Geometry: final body of the model. Coordinates: model frame, mm. A direction names the side the tool comes from. Coordinates: 2 decimals unless noted, no trailing zeros. Write each loop counter-clockwise with the first axis right and the second up, starting at its lowest first coordinate (ties: lowest second). Pieces come first, ordered by that corner, then holes.
from build123d import *

# Parameters (mm, degrees)
SKETCH_1_R               = 9.25
SKETCH_1_R_2             = 2.5
EXTRUDE_1_DEPTH          = 8
SKETCH_2_R               = 2.5
CUT_EXTRUDE_1_DEPTH      = 9
CUT_EXTRUDE_2_DEPTH      = 9
SKETCH_8_R               = 9.25
SKETCH_8_R_2             = 2.5
EXTRUDE_2_DEPTH          = 8
SKETCH_9_R               = 1.75
CUT_EXTRUDE_5_DEPTH      = 56
CUT_EXTRUDE_5_DEPTH_BACK = 56
SKETCH_11_W              = 2.84011948
SKETCH_11_H              = 7
CUT_EXTRUDE_6_DEPTH      = 8
EXTRUDE_3_DEPTH          = 8
SKETCH_12_R              = 1.65
CUT_EXTRUDE_7_DEPTH      = 9
CHAMFER_2_SIZE           = 1


with BuildPart() as part:
    # Sketch 1 → Extrude 1 (new body)
    with BuildSketch(Plane.XY):
        with BuildLine():
            Line((-50, -20), (50, -20))
            ThreePointArc((50, -20), (54.789131426, -16.436739428), (52.752293578, -10.825688073))
            Line((52.752293578, -10.825688073), (11.009174312, 16.697247706))
            ThreePointArc((11.009174312, 16.697247706), (0, 20), (-11.009174312, 16.697247706))
            Line((-11.009174312, 16.697247706), (-52.752293578, -10.825688073))
            ThreePointArc((-52.752293578, -10.825688073), (-54.789131426, -16.436739428), (-50, -20))
        make_face()
        Circle(SKETCH_1_R, mode=Mode.SUBTRACT)
        with Locations((50, -15)):
            Circle(SKETCH_1_R_2, mode=Mode.SUBTRACT)
        with Locations((-50, -15)):
            Circle(SKETCH_1_R_2, mode=Mode.SUBTRACT)
    extrude(amount=EXTRUDE_1_DEPTH)

    # Sketch 2 → Cut-Extrude 1 (cut, through all)
    with BuildSketch(Plane.XY.offset(8)):
        with Locations((0, 15)):
            Circle(SKETCH_2_R)
        with Locations((-10.606601718, 10.606601718)):
            Circle(SKETCH_2_R)
        with Locations((10.606601718, 10.606601718)):
            Circle(SKETCH_2_R)
    extrude(amount=-CUT_EXTRUDE_1_DEPTH, mode=Mode.SUBTRACT)

    # Sketch 3 → Cut-Extrude 2 (cut, through all)
    with BuildSketch(Plane.XY.offset(8)):
        with BuildLine():
            Line((-44.573394495, -11.422018349), (-15.198052695, 7.946338883))
            ThreePointArc((-15.198052695, 7.946338883), (-13.864095006, 6.417668929), (-12.053948035, 5.501348633))
            ThreePointArc((-12.053948035, 5.501348633), (-12.001148515, -5.615597414), (-3.5, -12.779377919))
            Line((-3.5, -12.779377919), (-3.5, -15))
            Line((-3.5, -15), (-43.5, -15))
            ThreePointArc((-43.5, -15), (-43.774129146, -13.132238744), (-44.573394495, -11.422018349))
        make_face()
    cut_extrude_2 = extrude(amount=-CUT_EXTRUDE_2_DEPTH, mode=Mode.SUBTRACT)

    # Mirror 1: Cut-Extrude 2 across plane
    add(cut_extrude_2.mirror(Plane(origin=(0, 0, 0), x_dir=(0, 0, 1), z_dir=(1, 0, 0))), mode=Mode.SUBTRACT)

    # Sketch 8 → Extrude 2 (add)
    with BuildSketch(Plane.XY.offset(8)):
        with BuildLine():
            Line((-11.009174312, 16.697247706), (-13.527583827, 15.036757916))
            ThreePointArc((-13.527583827, 15.036757916), (-15.771645109, 11.823461278), (-15.198052695, 7.946338883))
            ThreePointArc((-15.198052695, 7.946338883), (-13.864095006, 6.417668929), (-12.053948035, 5.501348633))
            ThreePointArc((-12.053948035, 5.501348633), (-12.001148515, -5.615597414), (-3.5, -12.779377919))
            ThreePointArc((-3.5, -12.779377919), (0, -13.25), (3.5, -12.779377919))
            ThreePointArc((3.5, -12.779377919), (12.001148515, -5.615597414), (12.053948035, 5.501348633))
            ThreePointArc((12.053948035, 5.501348633), (13.864095006, 6.417668929), (15.198052695, 7.946338883))
            ThreePointArc((15.198052695, 7.946338883), (15.771645109, 11.823461278), (13.527583827, 15.036757916))
            Line((13.527583827, 15.036757916), (11.009174312, 16.697247706))
            ThreePointArc((11.009174312, 16.697247706), (0, 20), (-11.009174312, 16.697247706))
        make_face()
        Circle(SKETCH_8_R, mode=Mode.SUBTRACT)
        with Locations((-10.606601718, 10.606601718)):
            Circle(SKETCH_8_R_2, mode=Mode.SUBTRACT)
        with Locations((10.606601718, 10.606601718)):
            Circle(SKETCH_8_R_2, mode=Mode.SUBTRACT)
        with Locations((0, 15)):
            Circle(SKETCH_8_R_2, mode=Mode.SUBTRACT)
    extrude(amount=EXTRUDE_2_DEPTH)

    # Sketch 9 → Cut-Extrude 5 (cut, two sides)
    with BuildSketch(Plane(origin=(0, 0, 0), x_dir=(0, 0, -1), z_dir=(1, 0, 0))) as cut_extrude_5_sk:
        with Locations((-12, 0)):
            Circle(SKETCH_9_R)
    extrude(amount=CUT_EXTRUDE_5_DEPTH, mode=Mode.SUBTRACT)
    extrude(cut_extrude_5_sk.sketch, amount=-CUT_EXTRUDE_5_DEPTH_BACK, mode=Mode.SUBTRACT)

    # Sketch 11 → Cut-Extrude 6 (cut)
    with BuildSketch(Plane.XY.offset(16)):
        with Locations((14.199437659, 0)):
            Rectangle(SKETCH_11_W, SKETCH_11_H)
        with Locations((-14.199437659, 0)):
            Rectangle(SKETCH_11_W, SKETCH_11_H)
    extrude(amount=-CUT_EXTRUDE_6_DEPTH, mode=Mode.SUBTRACT)

    # Sketch 13 → Extrude 3 (add)
    with BuildSketch(Plane.XY.offset(8)):
        with BuildLine():
            Line((-37.875, -10), (-35, -10))
            ThreePointArc((-35, -10), (-30, -15), (-35, -20))
            Line((-35, -20), (-44.573394495, -20))
            Line((-44.573394495, -20), (-44.573394495, -11.422018349))
            Line((-44.573394495, -11.422018349), (-39.251146789, -7.912844037))
            Line((-39.251146789, -7.912844037), (-37.875, -10))
        make_face()
    extrude_3 = extrude(amount=-EXTRUDE_3_DEPTH)

    # Sketch 12 → Cut-Extrude 7 (cut, through all)
    with BuildSketch(Plane.XY.offset(8)):
        with Locations((-42, -15)):
            Circle(SKETCH_12_R)
        with Locations((-35, -15)):
            Circle(SKETCH_12_R)
    cut_extrude_7 = extrude(amount=-CUT_EXTRUDE_7_DEPTH, mode=Mode.SUBTRACT)

    # Mirror 2: Extrude 3, Cut-Extrude 7 across plane
    add(extrude_3.mirror(Plane(origin=(0, 0, 0), x_dir=(0, 0, 1), z_dir=(1, 0, 0))))
    add(cut_extrude_7.mirror(Plane(origin=(0, 0, 0), x_dir=(0, 0, 1), z_dir=(1, 0, 0))), mode=Mode.SUBTRACT)

    # Chamfer 2
    chamfer_2_edges = [part.edges().sort_by_distance(p)[0] for p in [
        (8.106601718, 10.606601718, 0),
        (-13.106601718, 10.606601718, 0),
        (-2.5, 15, 0),
        (-13.106601718, 10.606601718, 16),
        (-2.5, 15, 16),
        (8.106601718, 10.606601718, 16),
    ]]
    chamfer(chamfer_2_edges, length=CHAMFER_2_SIZE)


solid = part.part
Item 1: Material intervals for probe 1 along Y at (x, z) = (0, 5.25); probe 2 along X at (y, z) = (-7, 3.25); probe 3 along Y at (x, z) = (9.95, 12), sorted ascending.
Derived:
probe 1: y = -20 to -9.25, 9.25 to 12.5, 17.5 to 20
probe 2: x = -46.95 to -37.87, -11.25 to -6.05, 6.05 to 11.25, 37.87 to 46.95
probe 3: y = -8.75 to -1.75, 1.75 to 8.19, 13.02 to 17.35
Item 2: Set-up query: faces 1 (the flat face through (-36, -10, 4)), 2 (the cylindrical face through (-10.905, 0.526, 10.331)). Return all of +Z, -Z, +X, -X, +Y, -Y with unobstructed straight access to the full face (end or side cutting, diameter ignored); none if empty.
Derived:
face 1: +Z, -Z
face 2: +X, -X
Item 3: Section A-A, the plane x = 0. Output: boundary loops of the cut face in (y, z).
Derived:
outline: (-20, 0) - (-9.25, 0) - (-9.25, 16) - (-13.25, 16) - (-13.25, 8) - (-20, 8) - close; (9.25, 0) - (11.5, 0) - (12.5, 1) - (12.5, 15) - (11.5, 16) - (9.25, 16) - close; (17.5, 1) - (18.5, 0) - (20, 0) - (20, 16) - (18.5, 16) - (17.5, 15) - close
Item 4: Pin query (flat end, axial travel): pin 1 (1 mm diameter, centred on y = 15, z = 8.5, fed in from +X); pin 2 (4 mm diameter, centred on x = 42, y = -15, fed in from +Z); pin 3 (2 mm diameter, centred on y = 0, z = 12, fed in from -X); pin 4 (1 mm diameter, centred on x = 31, y = -14, fed in from -Z). Return the tip coordinate at first contact, or that it passes through.
Derived:
pin 1: stops at x = 14.21
pin 2: stops at z = 8
pin 3: passes through
pin 4: stops at z = 0
Item 5: Section C-C, the plane x = 32. Output: boundary loops of the cut face in (y, z).
Derived:
outline: (-20, 0) - (-11, 0) - (-11, 8) - (-20, 8) - close; (-3.13, 0) - (2.86, 0) - (2.86, 8) - (-3.13, 8) - close
Item 6: Section D-D, the plane z = 5. State how many separate pieces and enclosed holes the cut face has, plus the area to 3 significant figures.
Derived:
separate pieces: 1
enclosed holes: 12
area: 1,560 mm2
Item 7: Pull-direction query (X, two-part tool) for faces 3 (the cylindrical face through (54.763, -16.522, 3.944)), 4 (the flat face through (-38.6, -8.9, 4.1)), 5 (the cylindrical face through (-54.8, -16.4, 3.9)); classes: released by +X, released by -X, zero draft, split by the parting line, or undercut.
Derived:
face 3: released by +X
face 4: undercut
face 5: released by -X
Item 8: Section B-B, the plane z = 12. Output: boundary loops of the cut face in (x, y), plus the area to 3 significant figures.
Derived:
outline: (-13.53, 15.04) arc R5.31 ccw to (-12.05, 5.5) arc R13.25 ccw to (-12.78, 3.5) - (-12.78, 1.75) - (-9.08, 1.75) arc R9.25 cw to (9.08, 1.75) - (12.78, 1.75) - (12.78, 3.5) arc R13.25 ccw to (12.05, 5.5) arc R5.31 ccw to (13.53, 15.04) - (11.01, 16.7) arc R20 ccw to (-11.01, 16.7) - close; (-12.78, -3.5) arc R13.25 ccw to (12.78, -3.5) - (12.78, -1.75) - (9.08, -1.75) arc R9.25 cw to (-9.08, -1.75) - (-12.78, -1.75) - close; hole circle Ø5 at (-10.61, 10.61); hole circle Ø5 at (0, 15); hole circle Ø5 at (10.61, 10.61)
area: 437 mm2
